Work out the finished part from the listing and answer in its coordinate system (mm). Face numbers are marked on the shaded views. A direction names the side the tool comes from. Round coordinates to 2 decimals unless told otherwise and drop trailing zeros. Write each loop counter-clockwise with the first axis right and the second up, starting at its lowest first coordinate (ties: lowest second). Pieces come first, ordered by that corner, then holes. Notation, with made-up numbers: M 0,0 L 56,0 A16 cw 56,13 Z; hole C 26,-21 d5. An arc over 180 degrees is marked long. Answer in a Markdown table with one row per item.
```python
from build123d import *

# Parameters (mm, degrees)
ESQUISSE1_W                                = 80
ESQUISSE1_H                                = 60
BOSS_EXTRU_1_DEPTH                         = 80
COQUE1_T                                   = -2.4
BOSS_EXTRU_2_REACH                         = 96.34
SYM_TRIE1_AT_THE_SECOND_PLANE_COPY_1_REACH = 96.34


with BuildPart() as part:
    # Esquisse1 → Boss.-Extru.1 (new body)
    with BuildSketch(Plane.XY):
        Rectangle(ESQUISSE1_W, ESQUISSE1_H)
    extrude(amount=BOSS_EXTRU_1_DEPTH)

    # Coque1
    coque1_openings = [part.faces().sort_by_distance(p)[0] for p in [
        (0, 0, 80),
    ]]
    offset(amount=COQUE1_T, openings=coque1_openings, kind=Kind.INTERSECTION)

    # Esquisse2 → Boss.-Extru.2 (add, up to next)
    with BuildSketch(Plane.XY.offset(80), mode=Mode.PRIVATE) as boss_extru_2_sk1:
        with BuildLine():
            Line((-37.6, 27.6), (-37.6, 19.6))
            ThreePointArc((-37.6, 19.6), (-31.943145751, 21.943145751), (-29.6, 27.6))
            Line((-29.6, 27.6), (-37.6, 27.6))
        make_face()
    boss_extru_2_tool1 = extrude(boss_extru_2_sk1.sketch, amount=-BOSS_EXTRU_2_REACH, mode=Mode.PRIVATE) - part.part
    boss_extru_2 = boss_extru_2_tool1.solids().sort_by_distance((-34.204695, 24.204695, 80))[0]
    add(boss_extru_2)

    # Esquisse4 → Dégagement M31 (revolve, cut)
    with BuildSketch(Plane(origin=(-35.488231032, 25.460651403, 80), x_dir=(0, -1, 0), z_dir=(1, 0, 0))):
        Polygon((0, 0), (0, 11.021463052), (1.7, 10), (1.7, 0), align=None)
    d_gagement_m31 = revolve(axis=Axis((-35.488231032, 25.460651403, 86.35), (0, 0, -1)), mode=Mode.SUBTRACT)

    # Symétrie1: Boss.-Extru.2, Dégagement M31 across plane
    add(boss_extru_2.mirror(Plane(origin=(0, 0, 0), x_dir=(0, 0, 1), z_dir=(1, 0, 0))))
    add(d_gagement_m31.mirror(Plane(origin=(0, 0, 0), x_dir=(0, 0, 1), z_dir=(1, 0, 0))), mode=Mode.SUBTRACT)

    # Symétrie1 at the second plane: Boss.-Extru.2, Dégagement M31 across plane
    add(boss_extru_2.mirror(Plane.ZX))
    add(d_gagement_m31.mirror(Plane.ZX), mode=Mode.SUBTRACT)

    # Symétrie1 at the second plane copy 1 ske → Symétrie1 at the second plane copy 1 (add, up to next)
    with BuildSketch(Plane(origin=(0, 0, 80), x_dir=(-1, 0, 0), z_dir=(0, 0, 1)), mode=Mode.PRIVATE) as sym_trie1_at_the_second_plane_copy_1_sk1:
        with BuildLine():
            Line((-37.6, 27.6), (-37.6, 19.6))
            ThreePointArc((-37.6, 19.6), (-31.943145751, 21.943145751), (-29.6, 27.6))
            Line((-29.6, 27.6), (-37.6, 27.6))
        make_face()
    sym_trie1_at_the_second_plane_copy_1_tool1 = extrude(sym_trie1_at_the_second_plane_copy_1_sk1.sketch, amount=-SYM_TRIE1_AT_THE_SECOND_PLANE_COPY_1_REACH, mode=Mode.PRIVATE) - part.part
    add(sym_trie1_at_the_second_plane_copy_1_tool1.solids().sort_by_distance((34.204695, -24.204695, 80))[0])

    # Symétrie1 at the second plane copy 2 ske → Symétrie1 at the second plane copy 2 (revolve, cut)
    with BuildSketch(Plane(origin=(35.488231032, -25.460651403, 80), x_dir=(0, 1, 0), z_dir=(-1, 0, 0))):
        Polygon((0, 0), (0, 11.021463052), (1.7, 10), (1.7, 0), align=None)
    revolve(axis=Axis((35.488231032, -25.460651403, 86.35), (0, 0, -1)), mode=Mode.SUBTRACT)


solid = part.part
```
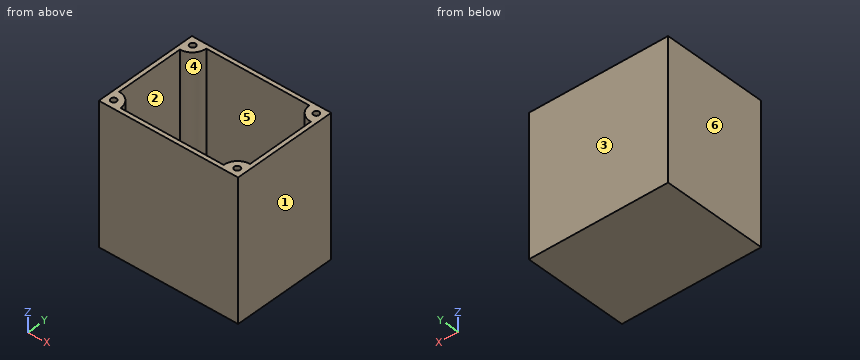
1. The part is cut by section C-C (y = 17). Determine the outline of the cut face in (x, z), plus the area to 3 significant figures.
Calculated:
| item | result |
|---|---|
| outline | M -40,0 L 40,0 L 40,80 L 37.6,80 L 37.6,2.4 L -37.6,2.4 L -37.6,80 L -40,80 Z |
| area | 564 mm² |
2. Determine the mould class of the marked faces 1, 2, 3 and 4 for opening direction X: released by +X, released by -X, zero draft, split by the parting line, or undercut.
Calculated:
| item | result |
|---|---|
| face 1 | released by +X |
| face 2 | undercut |
| face 3 | zero draft |
| face 4 | undercut |
3. The part is cut by section B-B (x = 11.5). Determine the outline of the cut face in (y, z), plus the area to 3 significant figures.
Calculated:
| item | result |
|---|---|
| outline | M -30,0 L 30,0 L 30,80 L 27.6,80 L 27.6,2.4 L -27.6,2.4 L -27.6,80 L -30,80 Z |
| area | 516 mm² |
4. The part is cut by section A-A (z = 65). Determine the outline of the cut face in (x, y).
Calculated:
| item | result |
|---|---|
| outline | M -40,-30 L 40,-30 L 40,30 L -40,30 Z; hole M -37.6,-19.6 A8 cw -29.6,-27.6 L 29.6,-27.6 A8 cw 37.6,-19.6 L 37.6,19.6 A8 cw 29.6,27.6 L -29.6,27.6 A8 cw -37.6,19.6 Z |
5. Given pin 1 (10 mm diameter, centred on x = -0.5, y = 20.5, fed in from +Z); pin 2 (2 mm diameter, centred on x = -35.49, y = -25.46, fed in from +Z), each flat-ended and moving along its own axis, determine where each tip first touches the part or whether it passes through.
Calculated:
| item | result |
|---|---|
| pin 1 | stops at z = 2.4 |
| pin 2 | stops at z = 69.58 |
6. Consider line 1 along X through (y, z) = (-13, 15.5); line 2 along Y through (x, z) = (-23.5, 66); line 3 along Z through (x, y) = (33.5, -20). Determine where each line is inside the solid, lowest interval first. Write a range as from..to.
Calculated:
| item | result |
|---|---|
| line 1 | x = -40..-37.6, 37.6..40 |
| line 2 | y = -30..-27.6, 27.6..30 |
| line 3 | z = 0..2.4 |
7. A tool of negligible diameter and unlimited length cuts with its end or side. For the marked faces 5 and 6, from which of +Z, -Z, +X, -X, +Y, -Y can it reach the whole face along a straight path? Write none if from no direction.
Calculated:
| item | result |
|---|---|
| face 5 | +Z |
| face 6 | +Z, -Z, -X, +Y, -Y |
